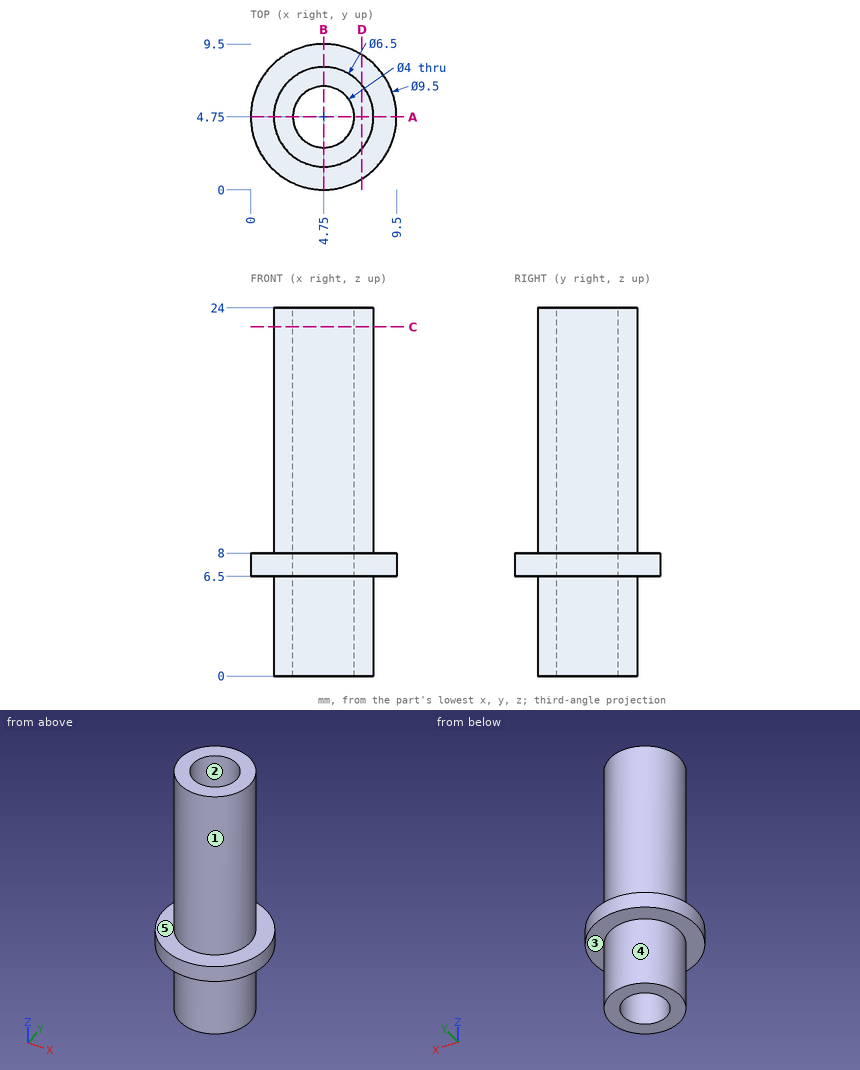
Input: dimensioned drawing with shaded views. Units: mm. Origin: part minimum x, y, z. A direction names the side the tool comes from. Coordinates: 2 decimals unless noted, no trailing zeros. Write each loop counter-clockwise with the first axis right and the second up, starting at its lowest first coordinate (ties: lowest second). Pieces come first, ordered by that corner, then holes. Notation, with made-up numbers: M 79.5,-24.5 L 92.5,-24.5 A16 ccw 92.5,-14.5 Z; hole C -0.75,-1.5 d11. An arc over 180 degrees is marked long. Answer as CSV lines item,"result". Start each with the question number.
Q1. Reachability of the marked faces 4 and 5 from +Z, -Z, +X, -X, +Y, -Y: full face, straight path, thin tool, end or side. Return the list, or none.
Q2. Line query: line 1 (X direction, y = 4.75, z = 19); line 2 (X direction, y = 4.75, z = 7.5). Output: solid intervals per line, ascending. Write a range as from..to.
Q3. Pin query (flat end, axial travel): P1, Ø4, axis at y = 2, z = 21.5, coming from the +X side; P2, Ø3.5, axis at x = 4.75, y = 4.75, coming from the +Z side; P3, Ø2, axis at x = 6, z = 12, coming from the +Y side; P4, Ø1.5, axis at x = 5.5, y = 8, coming from the -Z side. Return the tip coordinate at first contact, or that it passes through.
Q4. Cut plane A-A on y = 4.75. Return the cut outline in (x, z), then the cut area to 3 significant figures.
Q5. Cut plane D-D on x = 7.25. Return the cut outline in (y, z).
Q6. Mould query, pull axis X, two halves, no side actions, for the marked faces 1, 2 and 3. Classes: released by +X, released by -X, zero draft, split by the parting line, or undercut.
Q7. Cut plane C-C on z = 22.75. Return the cut outline in (x, y).
Findings below:
1,face 4,"-Z"
1,face 5,"+Z"
2,line 1,"x = 1.5..2.75, 6.75..8"
2,line 2,"x = 0..2.75, 6.75..9.5"
3,P1,"stops at x = 7.91"
3,P2,"passes through"
3,P3,"stops at y = 7.99"
3,P4,"stops at z = 0"
4,outline,"M 0,6.5 L 1.5,6.5 L 1.5,0 L 2.75,0 L 2.75,24 L 1.5,24 L 1.5,8 L 0,8 Z; M 6.75,0 L 8,0 L 8,6.5 L 9.5,6.5 L 9.5,8 L 8,8 L 8,24 L 6.75,24 Z"
4,area,"64.5 mm2"
5,outline,"M 0.71,6.5 L 2.67,6.5 L 2.67,0 L 6.83,0 L 6.83,6.5 L 8.79,6.5 L 8.79,8 L 6.83,8 L 6.83,24 L 2.67,24 L 2.67,8 L 0.71,8 Z"
6,face 1,"split by the parting line"
6,face 2,"undercut"
6,face 3,"zero draft"
7,outline,"C 4.75,4.75 d6.5; hole C 4.75,4.75 d4"
